Autodesk Inventor part; units mm, degrees
ref_plane "YZ Plane" through (0, 0, 0) normal (1, 0, 0) x (0, 1, 0)
ref_plane "XZ Plane" through (0, 0, 0) normal (0, 1, 0) x (-1, 0, 0)
ref_plane "XY Plane" through (0, 0, 0) normal (0, 0, 1) x (1, 0, 0)
sketch "Sketch1" plane through (0, 0, 0) normal (0, 0, 1) x (1, 0, 0)
  circle A0 centre (0, 0) radius 19.05
  dimension "d0" = 38.1
extrude "Extrusion1" add sketch "Sketch1" along normal blind 1.651
sketch "Sketch2" plane through (0, 0, 1.651) normal (0, 0, 1) x (1, 0, 0)
  circle A0 centre (0, 0) radius 19.05
  line L0 (-19.05, 19.05) -> (19.05, 19.05) construction
  line L1 (19.05, 19.05) -> (19.05, -19.05) construction
  line L2 (19.05, -19.05) -> (-19.05, -19.05) construction
  line L3 (-19.05, -19.05) -> (-19.05, 19.05) construction
  point P0 (0, 19.05)
  point P1 (-19.05, 0)
  point P2 (0, 19.05)
  point P3 (-19.05, 0)
decal "Decal1"
sketch "Sketch3" plane through (0, 0, 1.651) normal (0, 0, 1) x (1, 0, 0)
  circle A0 centre (-16.5947, 0) radius 1.397
  line L0 (19.05, -19.05) -> (-19.05, -19.05) construction
  line L1 (-19.05, -19.05) -> (-19.05, 19.05) construction
  line L2 (-19.05, 19.05) -> (19.05, 19.05) construction
  line L3 (19.05, 19.05) -> (19.05, -19.05) construction
  line L4 (19.05, -19.05) -> (-19.05, 19.05) construction
  line L5 (-19.05, -19.05) -> (19.05, 19.05) construction
  circle A1 centre (8.2973, 14.3714) radius 1.397
  circle A2 centre (8.2973, -14.3714) radius 1.397
  line L6 (-16.5947, 0) -> (8.2973, 14.3714) construction
  line L7 (8.2973, 14.3714) -> (8.2973, -14.3714) construction
  line L8 (8.2973, -14.3714) -> (-16.5947, 0) construction
  circle A3 centre (-2.54, 0) radius 0.6096
  circle A4 centre (2.54, 0) radius 0.6096
  point P0 (0, 0)
  point P1 (0, 0)
  dimension "d8" = 2.794
  dimension "d9" = 38.1
  dimension "d11" = 19.05
  dimension "d13" = 1.2192
  dimension "d14" = 5.08
  dimension "d15" = 2.54
  dimension "d25" = 24.892
  dimension "d26" = 2.4553
extrude "Extrusion2" cut sketch "Sketch3" against normal through all
sketch "Sketch5" plane through (0, 0, 0) normal (0, 0, -1) x (-1, 0, 0)
  circle A0 centre (0, 0) radius 19.05
  line L0 (-19.05, 19.05) -> (19.05, 19.05) construction
  line L1 (19.05, 19.05) -> (19.05, -19.05) construction
  line L2 (19.05, -19.05) -> (-19.05, -19.05) construction
  line L3 (-19.05, -19.05) -> (-19.05, 19.05) construction
  point P0 (-19.05, 0)
  point P1 (0, 19.05)
  point P2 (0, 19.05)
  point P3 (-19.05, 0)
decal "Decal3"
properties part number "Filament Board"
Build history of the part. All positions in model axes, mm. Round coordinates to 2 decimals unless told otherwise and drop trailing zeros. Order: outer loops, then holes, each group sorted by start corner. A loop starts at its lowest first (then second) coordinate and runs counter-clockwise, first axis right, second up. Notation, with made-up numbers: M 74,60 L 87,60 A12 ccw 87,66 Z; hole C 64.25,-32 d5. An arc over 180 degrees is marked long. Use CSV: the item, a comma, the result in double quotes. Start each with the question number.
(1) Cut at D-D on z = 1.1. List the corners of the cut face in (x, y).
(2) Drill centre lines: probe 1 along Y at (x, z) = (-16, 1.2); probe 2 along Y at (x, z) = (-2.54, 0.45); probe 3 along Y at (x, z) = (-0.5, 0.3). Where is each one in solid material? Low to high.
(3) Cut at C-C on y = -15. List the corners of the cut face in (x, z).
(4) Cut at A-A on y = 0. List the corners of the cut face in (x, z), then the cut area to 3 significant figures.
(5) Mould opens along Y. For faces 1 (the face through (9.63, 14.79, 0.84)), 2 (the face through (-15.12, 11.59, 0.81)), 3 (the face through (0, 0, 1.651)) say: +Y half, -Y half, draft (parallel to the pull), parting line (faces both ways), or undercut.
(6) Cut at B-B on x = -2.54. List the corners of the cut face in (y, z).
(7) Flat gauge pin, fed straight in: P1, Ø4.5, axis at x = 8.3, y = -14.37, coming from the +Z side. Where does the tip first touch, or does it go through?
Findings:
1,outline,"C 0,0 d38.1; hole C -16.59,0 d2.79; hole C -2.54,0 d1.22; hole C 2.54,0 d1.22; hole C 8.3,-14.37 d2.79; hole C 8.3,14.37 d2.79"
2,probe 1,"y = -10.34 to -1.26, 1.26 to 10.34"
2,probe 2,"y = -18.88 to -0.61, 0.61 to 18.88"
2,probe 3,"y = -19.04 to 19.04"
3,outline,"M -11.74,0 L 7.05,0 L 7.05,1.65 L -11.74,1.65 Z; M 9.54,0 L 11.74,0 L 11.74,1.65 L 9.54,1.65 Z"
4,outline,"M -19.05,0 L -17.99,0 L -17.99,1.65 L -19.05,1.65 Z; M -15.2,0 L -3.15,0 L -3.15,1.65 L -15.2,1.65 Z; M -1.93,0 L 1.93,0 L 1.93,1.65 L -1.93,1.65 Z; M 3.15,0 L 19.05,0 L 19.05,1.65 L 3.15,1.65 Z"
4,area,"54.3 mm^2"
5,face 1,"undercut"
5,face 2,"parting line"
5,face 3,"draft"
6,outline,"M -18.88,0 L -0.61,0 L -0.61,1.65 L -18.88,1.65 Z; M 0.61,0 L 18.88,0 L 18.88,1.65 L 0.61,1.65 Z"
7,P1,"stops at z = 1.65"
